Check sheet for the modelled part. Datum: model origin and axes. Units: mm. Face numbers are marked on the shaded views. Coordinates: 2 decimals unless noted, no trailing zeros. Write each loop counter-clockwise with the first axis right and the second up, starting at its lowest first coordinate (ties: lowest second). Pieces come first, ordered by that corner, then holes. Notation, with made-up numbers: M -0.75,62 L 4.25,62 A23 ccw 4.25,87 Z; hole C 44.25,-4.5 d8. An arc over 180 degrees is marked long. Answer as CSV lines item,"result". Start each with the question number.
Q1. Sectioned sample at A-A, the plane z = 5.75. Record the cut outline in (x, y), then the cut area to 3 significant figures.
Q2. Thickness scan on line 1 along Y through (x, z) = (0, 7.5); line 2 along Y through (x, z) = (-2, 5.5); line 3 along X through (y, z) = (1.5, 10.5). Record the ranges inside material, lowest first. Write a range as from..to.
Q3. Sectioned sample at B-B, the plane z = 12.5. Record the cut outline in (x, y), then the cut area to 3 significant figures.
Q4. Mould release check, pull along Y, two halves, no side actions. Record for the marked faces 1, 2 and 3: pulls with the +Y half, pulls with the -Y half, needs draft (parallel to the pull), parting line crosses it, or undercut.
Q5. Depth check by flat-ended pin: pin 1 Ø1 at (y, z) = (-3, 3.5) entering from +X; pin 2 Ø1.5 at (y, z) = (-5.5, 7) entering from +X; pin 3 Ø5 at (y, z) = (4.5, 3) entering from +X. Enter the tip coordinate at first touch or a pass-through.
Q6. Sectioned sample at C-C, the plane z = 10.75. Record the cut outline in (x, y).
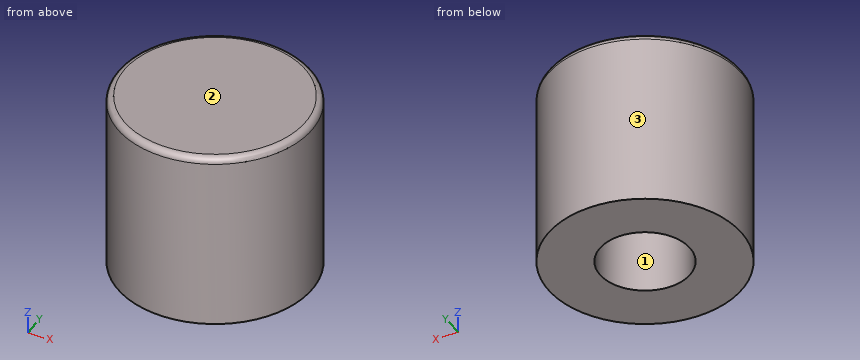
from build123d import *

# Parameters (mm, degrees)
SKETCH1_R                 = 7.5
BOSS_EXTRUDE1_DEPTH       = 14
M8X1_0_TAPPED_HOLE1_D     = 7
M8X1_0_TAPPED_HOLE1_DEPTH = 10
M8X1_0_TAPPED_HOLE1_TIP   = 2.020725942
FILLET1_R                 = 0.5


with BuildPart() as part:
    # Sketch1 → Boss-Extrude1 (new body)
    with BuildSketch(Plane.XY):
        Circle(SKETCH1_R)
    extrude(amount=BOSS_EXTRUDE1_DEPTH)

    # M8x1.0 Tapped Hole1
    with Locations(Plane(origin=(0, 0, 0), x_dir=(-1, 0, 0), z_dir=(0, 0, -1))):
        with Locations((0, 0)):
            Hole(M8X1_0_TAPPED_HOLE1_D / 2, depth=M8X1_0_TAPPED_HOLE1_DEPTH)
            with Locations((0, 0, -(M8X1_0_TAPPED_HOLE1_DEPTH + M8X1_0_TAPPED_HOLE1_TIP / 2))):  # 120° drill point
                Cone(0, M8X1_0_TAPPED_HOLE1_D / 2, M8X1_0_TAPPED_HOLE1_TIP, mode=Mode.SUBTRACT)

    # Fillet1
    fillet1_edges = [part.edges().sort_by_distance(p)[0] for p in [
        (-7.5, 0, 14),
    ]]
    fillet(fillet1_edges, radius=FILLET1_R)


solid = part.part
Output:
1,outline,"C 0,0 d15; hole C 0,0 d7"
1,area,"138 mm^2"
2,line 1,"y = -7.5..-3.5, 3.5..7.5"
2,line 2,"y = -7.23..-2.87, 2.87..7.23"
2,line 3,"x = -7.35..-2.17, 2.17..7.35"
3,outline,"C 0,0 d15"
3,area,"177 mm^2"
4,face 1,"undercut"
4,face 2,"needs draft"
4,face 3,"parting line crosses it"
5,pin 1,"stops at x = 7.07"
5,pin 2,"stops at x = 5.8"
5,pin 3,"stops at x = 7.23"
6,outline,"C 0,0 d15; hole C 0,0 d4.4"
